from build123d import *

# Parameters (mm, degrees)
F0_W     = 54
F0_H     = 76
F1_DEPTH = 2


with BuildPart() as f1:
    # F0 (on Top) → F1 (new body)
    with BuildSketch(Plane.XY):
        with Locations((-7.570542, 6.766017)):
            Rectangle(F0_W, F0_H)
        with BuildLine():
            ThreePointArc((-31.570542, 37.766017), (-30.398969, 40.594444), (-27.570542, 41.766017))
            Line((-27.570542, 41.766017), (12.429458, 41.766017))
            ThreePointArc((12.429458, 41.766017), (15.257886, 40.594444), (16.429458, 37.766017))
            Line((16.429458, 37.766017), (16.429458, -24.233983))
            ThreePointArc((16.429458, -24.233983), (15.257886, -27.062411), (12.429458, -28.233983))
            Line((12.429458, -28.233983), (-27.570542, -28.233983))
            ThreePointArc((-27.570542, -28.233983), (-30.398969, -27.062411), (-31.570542, -24.233983))
            Line((-31.570542, -24.233983), (-31.570542, 37.766017))
        make_face(mode=Mode.SUBTRACT)
    extrude(amount=F1_DEPTH)


solid = f1.part
The listing builds one solid part. Answer for the finished solid, in the listing's coordinates (mm). A direction names the side the tool comes from. Round coordinates to 2 decimals unless told otherwise and drop trailing zeros. Write each loop counter-clockwise with the first axis right and the second up, starting at its lowest first coordinate (ties: lowest second). Pieces come first, ordered by that corner, then holes. Notation, with made-up numbers: (-15, 59) - (11, 59) arc R35 cw to (11, 94) - close; hole circle Ø4 at (31, -12). An arc over 180 degrees is marked (long way). Use a Markdown table: item, result. Add a question column.
1. The part is cut by section B-B (y = -6). Write down the section's boundary in (x, z), and give its area (3 significant figures).
2. The part is cut by section A-A (x = -17). Write down the section's boundary in (y, z), and give its area (3 significant figures).
3. For a pull along X with two mould halves and no side action, classify faces 3 (the face through (19.429, 6, 1)), 4 (the face through (-8, -31.234, 1)), 5 (the face through (15.227, 40.625, 0.986)) as +X half, -X half, draft (parallel to the pull), parting line (faces both ways), or undercut.
4. Consider line 1 (Y direction, x = -13, z = 0.45); line 2 (X direction, y = -15, z = 1.7); line 3 (X direction, y = 41, z = 0.1). Determine where each line is inside the solid, lowest interval first.
5. A tool of negligible diameter and unlimited length cuts with its end or side. For faces 1 (the face through (15.29, -27.03, 0.99)), 2 (the face through (-32, 7, 2)), from which of +Z, -Z, +X, -X, +Y, -Y can it reach the whole face along a straight path? Write none if from no direction.
6. The part is cut by section C-C (z = 1.7). Write down the section's boundary in (x, y), and give its area (3 significant figures).
Reported:
| question | item | result |
|---|---|---|
| 1 | outline | (-34.57, 0) - (-31.57, 0) - (-31.57, 2) - (-34.57, 2) - close; (16.43, 0) - (19.43, 0) - (19.43, 2) - (16.43, 2) - close |
| 1 | area | 12.0 mm^2 |
| 2 | outline | (-31.23, 0) - (-28.23, 0) - (-28.23, 2) - (-31.23, 2) - close; (41.77, 0) - (44.77, 0) - (44.77, 2) - (41.77, 2) - close |
| 2 | area | 12.0 mm^2 |
| 3 | face 3 | +X half |
| 3 | face 4 | draft |
| 3 | face 5 | undercut |
| 4 | line 1 | -31.23 to -28.23, 41.77 to 44.77 |
| 4 | line 2 | -34.57 to -31.57, 16.43 to 19.43 |
| 4 | line 3 | -34.57 to -29.92, 14.78 to 19.43 |
| 5 | face 1 | +Z, -Z |
| 5 | face 2 | +Z, +X, -X, +Y, -Y |
| 6 | outline | (-34.57, -31.23) - (19.43, -31.23) - (19.43, 44.77) - (-34.57, 44.77) - close; hole (-31.57, -24.23) arc R4 ccw to (-27.57, -28.23) - (12.43, -28.23) arc R4 ccw to (16.43, -24.23) - (16.43, 37.77) arc R4 ccw to (12.43, 41.77) - (-27.57, 41.77) arc R4 ccw to (-31.57, 37.77) - close |
| 6 | area | 758 mm^2 |
